Source: CAD feature listing. Evaluate the final solid. Frame: model axes, mm. Give positions to 0.01 mm unless a question says otherwise; leave off trailing zeros. Order: outer loops, then holes, each group sorted by start corner. A loop starts at its lowest first (then second) coordinate and runs counter-clockwise, first axis right, second up. Notation, with made-up numbers: (-5, -39.75) - (16, -39.75) arc R27 cw to (16, -21.75) - close; hole circle Ø8 at (77, 68). An arc over 180 degrees is marked (long way). Write each question's results on one line, items separated by ' | '. Start each with the question number.
Item 1: Mould query, pull axis X, two halves, no side actions, for faces 1 (the flat face through (27, -27, 4)), 2 (the cylindrical face through (123.997, 39.048, 1.972)), 3 (the cylindrical face through (31, 9.76, 1.97)). Classes: released by +X, released by -X, zero draft, split by the parting line, or undercut.
Item 2: Section D-D on x = 100. Output: boundary loops of the cut face in (y, z), and give its area (3 significant figures).
Item 3: Section A-A on y = 0. Output: boundary loops of the cut face in (x, z).
Item 4: Contact query for flat-ended pins moving along their axis: pin 1 Ø1.5 at (y, z) = (-92, 1.5) entering from -X; pin 2 Ø1 at (y, z) = (-62.5, 1.5) entering from +X; pin 3 Ø1 at (y, z) = (-85.5, 3) entering from -X. Output: stop coordinate, or through.
Item 5: Line query: line 1 along X through (y, z) = (-90.5, 3.7); line 2 along Y through (x, z) = (100, 1.7); line 3 along Y through (x, z) = (-14, 3.85). Output: solid intervals per line, ascending.
Item 6: Section B-B on x = -50. Output: boundary loops of the cut face in (y, z), and give its area (3 significant figures).
```python
from build123d import *

# Parameters (mm, degrees)
SKETCH_1_R      = 130
SKETCH_1_R_2    = 32.5
SKETCH_1_R_3    = 5
SKETCH_1_R_4    = 1.6
EXTRUDE_1_DEPTH = 4


with BuildPart() as part:
    # 草图1 → 凸台-拉伸1 (new body)
    with BuildSketch(Plane.XY):
        Circle(SKETCH_1_R)
        Circle(SKETCH_1_R_2, mode=Mode.SUBTRACT)
        with Locations((0, 100)):
            Circle(SKETCH_1_R_3, mode=Mode.SUBTRACT)
        with Locations((50, 86.602540378)):
            Circle(SKETCH_1_R_3, mode=Mode.SUBTRACT)
        with Locations((86.602540378, 50)):
            Circle(SKETCH_1_R_3, mode=Mode.SUBTRACT)
        with Locations((100, 0)):
            Circle(SKETCH_1_R_3, mode=Mode.SUBTRACT)
        with Locations((86.602540378, -50)):
            Circle(SKETCH_1_R_3, mode=Mode.SUBTRACT)
        with Locations((50, -86.602540378)):
            Circle(SKETCH_1_R_3, mode=Mode.SUBTRACT)
        with Locations((0, -100)):
            Circle(SKETCH_1_R_3, mode=Mode.SUBTRACT)
        with Locations((-50, -86.602540378)):
            Circle(SKETCH_1_R_3, mode=Mode.SUBTRACT)
        with Locations((-86.602540378, -50)):
            Circle(SKETCH_1_R_3, mode=Mode.SUBTRACT)
        with Locations((-100, 0)):
            Circle(SKETCH_1_R_3, mode=Mode.SUBTRACT)
        with Locations((-86.602540378, 50)):
            Circle(SKETCH_1_R_3, mode=Mode.SUBTRACT)
        with Locations((-50, 86.602540378)):
            Circle(SKETCH_1_R_3, mode=Mode.SUBTRACT)
        with Locations((0, 44.5)):
            Circle(SKETCH_1_R_4, mode=Mode.SUBTRACT)
        with Locations((38.538130468, 22.25)):
            Circle(SKETCH_1_R_4, mode=Mode.SUBTRACT)
        with Locations((38.538130468, -22.25)):
            Circle(SKETCH_1_R_4, mode=Mode.SUBTRACT)
        with Locations((0, -44.5)):
            Circle(SKETCH_1_R_4, mode=Mode.SUBTRACT)
        with Locations((-38.538130468, -22.25)):
            Circle(SKETCH_1_R_4, mode=Mode.SUBTRACT)
        with Locations((-38.538130468, 22.25)):
            Circle(SKETCH_1_R_4, mode=Mode.SUBTRACT)
    extrude(amount=EXTRUDE_1_DEPTH)


solid = part.part
```
Evaluation:
1) face 1: zero draft | face 2: split by the parting line | face 3: undercut
2) outline: (-83.07, 0) - (-5, 0) - (-5, 4) - (-83.07, 4) - close; (5, 0) - (83.07, 0) - (83.07, 4) - (5, 4) - close | area: 625 mm^2
3) outline: (-130, 0) - (-105, 0) - (-105, 4) - (-130, 4) - close; (-95, 0) - (-32.5, 0) - (-32.5, 4) - (-95, 4) - close; (32.5, 0) - (95, 0) - (95, 4) - (32.5, 4) - close; (105, 0) - (130, 0) - (130, 4) - (105, 4) - close
4) pin 1: stops at x = -92.59 | pin 2: stops at x = 114.26 | pin 3: stops at x = -98.36
5) line 1: x = -93.33 to -53.13, -46.87 to 46.87, 53.13 to 93.33 | line 2: y = -83.07 to -5, 5 to 83.07 | line 3: y = -129.24 to -29.33, 29.33 to 129.24
6) outline: (-120, 0) - (-91.6, 0) - (-91.6, 4) - (-120, 4) - close; (-81.6, 0) - (81.6, 0) - (81.6, 4) - (-81.6, 4) - close; (91.6, 0) - (120, 0) - (120, 4) - (91.6, 4) - close | area: 880 mm^2
